from build123d import *

# Parameters (mm, degrees)
SKETCH_4_W          = 32
SKETCH_4_H          = 15.5
EXTRUDE_2_DEPTH     = 20
SKETCH_6_W          = 23
SKETCH_6_H          = 12.5
CUT_EXTRUDE_1_DEPTH = 27.759344162
CUT_EXTRUDE_2_REACH = 40.524
SKETCH_7_W          = 4
SKETCH_7_H          = 11
SKETCH_9_R          = 1.35
CUT_EXTRUDE_3_DEPTH = 10
SKETCH_11_R         = 2.1
CUT_EXTRUDE_4_DEPTH = 5


with BuildPart() as part:
    # Эскиз4 → Бобышка-Вытянуть2 (new body)
    with BuildSketch(Plane.XY):
        Rectangle(SKETCH_4_W, SKETCH_4_H)
    extrude(amount=EXTRUDE_2_DEPTH)

    # Эскиз6 → Вырез-Вытянуть1 (cut, through all)
    with BuildSketch(Plane(origin=(0, 0, 0), x_dir=(-1, 0, 0), z_dir=(0, 0, -1))):
        with Locations((0, 1.5)):
            Rectangle(SKETCH_6_W, SKETCH_6_H)
    extrude(amount=-CUT_EXTRUDE_1_DEPTH, mode=Mode.SUBTRACT)

    # Эскиз7 → Вырез-Вытянуть2 (cut, up to next)
    with BuildSketch(Plane.ZY.offset(16), mode=Mode.PRIVATE) as cut_extrude_2_sk1:
        with Locations((8, 2.25)):
            Rectangle(SKETCH_7_W, SKETCH_7_H)
    cut_extrude_2_tool1 = extrude(cut_extrude_2_sk1.sketch, amount=-CUT_EXTRUDE_2_REACH, mode=Mode.PRIVATE) & part.part
    add(cut_extrude_2_tool1.solids().sort_by_distance((-16, 2.25, 8))[0], mode=Mode.SUBTRACT)

    # Эскиз9 → Вырез-Вытянуть3 (cut)
    with BuildSketch(Plane.XY.offset(20)):
        with Locations((-14.3, 1.25)):
            Circle(SKETCH_9_R)
        with Locations((14.3, 1.25)):
            Circle(SKETCH_9_R)
    extrude(amount=-CUT_EXTRUDE_3_DEPTH, mode=Mode.SUBTRACT)

    # Эскиз11 → Вырез-Вытянуть4 (cut)
    with BuildSketch(Plane.XZ.offset(7.75)):
        with Locations(Location((-10, 15, 0), (0, 0, 270))):
            Circle(SKETCH_11_R)
        with Locations(Location((10, 15, 0), (0, 0, 270))):
            Circle(SKETCH_11_R)
        with Locations(Location((10, 5, 0), (0, 0, 270))):
            Circle(SKETCH_11_R)
        with Locations(Location((-10, 5, 0), (0, 0, 270))):
            Circle(SKETCH_11_R)
    extrude(amount=-CUT_EXTRUDE_4_DEPTH, mode=Mode.SUBTRACT)


solid = part.part
Model file for the job. Use its own axes, mm. A direction names the side the tool comes from. Coordinates: 2 decimals unless noted, no trailing zeros. Write each loop counter-clockwise with the first axis right and the second up, starting at its lowest first coordinate (ties: lowest second). Pieces come first, ordered by that corner, then holes. Notation, with made-up numbers: (55, 28) -> (63, 28) arc R18 ccw to (63, 42) -> close; hole circle Ø8 at (-31, 40.25). An arc over 180 degrees is marked (long way). One line per item, written item: value. Start each with the question number.
1) Slice it at B-B on x = -14.3. Write the cut outline in (y, z), then the cut area to 3 significant figures.
2) Flat gauge pins, fed straight in: pin 1 Ø2 at (x, y) = (-14.3, 1.25) entering from +Z; pin 2 Ø3.5 at (x, z) = (-10, 5) entering from -Y; pin 3 Ø5 at (x, y) = (-11, -4) entering from +Z; pin 4 Ø6 at (x, z) = (-3.5, 10) entering from +Y. Where does each tip first touch, or does it go through?
3) Pull direction Y, two halves, no side cores. Call faces 5 (the face through (14, 1, 10)), 6 (the face through (-11.5, 1, 15)), 7 (the face through (-14, -3.25, 8)): +Y half, -Y half, draft (parallel to the pull), parting line (faces both ways), or undercut.
4) Slice it at C-C on y = 1.25. Write the cut outline in (x, z).
5) Which spindle directions (+Z, -Z, +X, -X, +Y, -Y) get a long thin tool onto all of the face, cutting with end or side? Do faces 1 (the face through (-12.05, -5.84, 15.46)), 2 (the face through (-13.053, 0.733, 15.07)), 3 (the face through (-14, 2, 6)), 4 (the face through (11.5, 1, 10)). Say none if no direction does.
6) Slice it at D-D on x = 10. Write the cut outline in (y, z), then the cut area to 3 significant figures.
7) Probe probe 1 along Z at (x, y) = (10, -5.3); probe 2 along X at (y, z) = (-5.7, 15); probe 3 along X at (y, z) = (-0.5, 5.5). List the from-to ranges inside material, lowest first.
8) Slice it at A-A on z = 5. Write the cut outline in (x, y).
Answers follow:
1. outline: (-7.75, 0) -> (7.75, 0) -> (7.75, 6) -> (-3.25, 6) -> (-3.25, 10) -> (-0.1, 10) -> (-0.1, 20) -> (-7.75, 20) -> close; (2.6, 10) -> (7.75, 10) -> (7.75, 20) -> (2.6, 20) -> close
1. area: 239 mm2
2. pin 1: z = 6
2. pin 2: y = -2.75
2. pin 3: z = 20
2. pin 4: y = -4.75
3. face 5: undercut
3. face 6: draft
3. face 7: +Y half
4. outline: (-16, 0) -> (-11.5, 0) -> (-11.5, 6) -> (-16, 6) -> close; (-16, 10) -> (-15.65, 10) -> (-15.65, 20) -> (-16, 20) -> close; (-12.95, 10) -> (-11.5, 10) -> (-11.5, 20) -> (-12.95, 20) -> close; (11.5, 0) -> (16, 0) -> (16, 20) -> (15.65, 20) -> (15.65, 10) -> (12.95, 10) -> (12.95, 20) -> (11.5, 20) -> close
5. face 1: -Y
5. face 2: +Z
5. face 3: -X, +Y
5. face 4: +Z, -Z, +Y
6. outline: (-7.75, 0) -> (-4.75, 0) -> (-4.75, 2.9) -> (-7.75, 2.9) -> close; (-7.75, 7.1) -> (-4.75, 7.1) -> (-4.75, 12.9) -> (-7.75, 12.9) -> close; (-7.75, 17.1) -> (-4.75, 17.1) -> (-4.75, 20) -> (-7.75, 20) -> close
6. area: 34.8 mm2
7. probe 1: 0 to 2.9, 7.1 to 12.9, 17.1 to 20
7. probe 2: -16 to -12.1, -7.9 to 7.9, 12.1 to 16
7. probe 3: -16 to -11.5, 11.5 to 16
8. outline: (-16, -7.75) -> (-12.1, -7.75) -> (-12.1, -2.75) -> (-11.5, -2.75) -> (-11.5, 7.75) -> (-16, 7.75) -> close; (-7.9, -7.75) -> (7.9, -7.75) -> (7.9, -4.75) -> (-7.9, -4.75) -> close; (11.5, -2.75) -> (12.1, -2.75) -> (12.1, -7.75) -> (16, -7.75) -> (16, 7.75) -> (11.5, 7.75) -> close
